```python
from build123d import *

# Parameters (mm, degrees)
F0_R        = 7.874
F1_DEPTH    = 10.922
F0_W        = 52.578
F0_H        = 10.922
F2_DEPTH    = 33.528
F3_SIZE2    = 22.1192058352
F3_SIZE     = 82.55
F4_T4_DEPTH = 283.7447130195
F5_SIZE2    = 16.5711074263
F5_SIZE     = 28.702


# Not quite as in the source:
# - a fillet or chamfer that OpenCascade refuses, or shapes differently, is made with other operations: its cross-section is extruded or revolved along the edge and cut away or added


with BuildPart() as f1:
    # F0 (on Front) → F1 (new body)
    with BuildSketch(Plane.XZ):
        Polygon((56.9204140842, 23.2569413837), (-57.3795859158, 23.2569413837), (-57.3795859158, 13.8589413837), (-46.4575859158, 13.8589413837), (-46.4575859158, -26.0190586163), (6.1204140842, -26.0190586163), (6.1204140842, -36.9410586163), (56.9204140842, -36.9410586163), align=None)
        with Locations((37.8704140842, -17.8910586163)):
            Circle(F0_R, mode=Mode.SUBTRACT)
    extrude(amount=F1_DEPTH)

    # F0 (on Front) → F2 (join)
    with BuildSketch(Plane.XZ):
        Polygon((-46.4575859158, 13.8589413837), (-57.3795859158, 13.8589413837), (-57.3795859158, -36.9410586163), (-46.4575859158, -36.9410586163), (-46.4575859158, -26.0190586163), align=None)
        with Locations((-20.1685859158, -31.4800586163)):
            Rectangle(F0_W, F0_H)
    extrude(amount=F2_DEPTH)

    # F3
    f3_edges = [f1.edges().sort_by_distance(p)[0] for p in [
        (56.920414, -5.461, 23.256941),
    ]]
    f3_side = f1.faces().sort_by_distance((-0.229586, -5.461, 23.256941))[0]
    chamfer(f3_edges, length=F3_SIZE, length2=F3_SIZE2, reference=f3_side)

    # F4: chamfer of 25.4 x 52.6596501835 on 1 edges, made by hand


with BuildPart() as f4_tool2:
    # F4_s3 → F4_t4 (new body)
    with BuildSketch(Plane.XY.offset(-173.3524151261)):
        Polygon((-46.5392360993, -33.528), (6.1204140842, -8.128), (6.1204140842, -33.528), align=None)
    extrude(amount=F4_T4_DEPTH)

    split(bisect_by=Plane.XZ.offset(10.922), keep=Keep.TOP)


with BuildPart() as f1_1:
    add(f1.part)

    # F4_t1: cut F4_tool2
    add(f4_tool2.part, mode=Mode.SUBTRACT)

    # F5
    f5_edges = [f1_1.edges().sort_by_distance(p)[0] for p in [
        (-51.959411, -33.528, 13.858941),
    ]]
    f5_side = f1_1.faces().sort_by_distance((-51.959411, -33.528, -11.541059))[0]
    chamfer(f5_edges, length=F5_SIZE, length2=F5_SIZE2, reference=f5_side)


solid = f1_1.part
```
Input: part model. Units: mm. Frame: model coordinates. A direction names the side the tool comes from. Give positions to 0.01 mm unless a question says otherwise; leave off trailing zeros. Order: outer loops, then holes, each group sorted by start corner. A loop starts at its lowest first (then second) coordinate and runs counter-clockwise, first axis right, second up. Notation, with made-up numbers: (10, 52.25) - (15, 52.25) arc R9 ccw to (15, 66.25) - close; hole circle Ø2 at (-20, 53). An arc over 180 degrees is marked (long way). Put each result on its own line as item: value.
Item 1: Section query C-C, the plane y = -3. Return loops of the section in (x, z).
Found:
outline: (-57.38, -36.94) - (56.92, -36.94) - (56.92, 1.14) - (-25.63, 23.26) - (-57.38, 23.26) - close; hole circle Ø15.75 at (37.87, -17.89)
Item 2: Section query A-A, the plane z = -23. Return loops of the section in (x, y), then the cut area to 3 significant figures.
Found:
outline: (-57.38, -33.53) - (-46.54, -33.53) - (-46.46, -33.49) - (-46.46, -10.92) - (31.88, -10.92) - (31.88, 0) - (-57.38, 0) - close; (43.86, -10.92) - (56.92, -10.92) - (56.92, 0) - (43.86, 0) - close
area: 1,360 mm^2
Item 3: Access query for faces 5 (the flat face through (-29, -20, -26.019)), 6 (the flat face through (-52, -33.528, -26)). Directions: +Z, -Z, +X, -X, +Y, -Y. A direction counts if a zero-diameter tool reaches every point of the face in a straight line with its end or side. Return the directions, or none.
Found:
face 5: +Z, +X, -Y
face 6: +Z, -Z, +X, -X, -Y
Item 4: Section query D-D, the plane x = -14.5. Return loops of the section in (y, z).
Found:
outline: (-18.07, -36.94) - (0, -36.94) - (0, 20.27) - (-10.92, 20.27) - (-10.92, -26.02) - (-18.07, -26.02) - close
Item 5: Section query B-B, the plane x = 42. Return loops of the section in (y, z).
Found:
outline: (-10.92, -36.94) - (0, -36.94) - (0, -24.6) - (-10.92, -24.6) - close; (-10.92, -11.19) - (0, -11.19) - (0, 5.14) - (-10.92, 5.14) - close
Item 6: Contact query for flat-ended pins moving along their axis: pin 1 (2 mm diameter, centred on x = -10.5, z = -4, fed in from -Y); pin 2 (10 mm diameter, centred on x = 33.5, z = 13.5, fed in from -Y); pin 3 (11.5 mm diameter, centred on x = -32, y = -23.5, fed in from +Z); pin 4 (1.8 mm diameter, centred on x = -50, y = -15, fed in from +Z). Output: stop coordinate, or through.
Found:
pin 1: stops at y = -10.92
pin 2: passes through
pin 3: stops at z = -26.02
pin 4: stops at z = 13.86
Item 7: Ray query, L1, parallel to Y at x = -29.5, z = -23.5; L2, parallel to X at y = -29, z = -16.5; L3, parallel to X at y = -4.5, z = -20. Return the intervals inside material, ascending. Write a range as from..to.
Found:
L1: y = -10.92..0
L2: x = -57.38..-46.46
L3: x = -57.38..30.28, 45.46..56.92
Item 8: Draft query along Z for faces 1 (the flat face through (-1, 0, -13)), 2 (the flat face through (-52, -14, 13.859)), 3 (the cylindrical face through (36.163, -5.385, -25.578)), 4 (the flat face through (-14, -9, -36.941)). Return one class per face: +Z half, -Z half, draft (parallel to the pull), parting line (faces both ways), or undercut.
Found:
face 1: draft
face 2: +Z half
face 3: undercut
face 4: -Z half
